Could you check a few things on this model? Use its own coordinates, in mm. A direction names the side the tool comes from. Round coordinates to 2 decimals unless told otherwise and drop trailing zeros. Write each loop counter-clockwise with the first axis right and the second up, starting at its lowest first coordinate (ties: lowest second). Pieces come first, ordered by that corner, then holes. Notation, with made-up numbers: (-40, 47.5) -> (-9, 47.5) arc R21 cw to (-9, 81.5) -> close; hole circle Ø1 at (84, 74.25). An arc over 180 degrees is marked (long way). Answer in a Markdown table with one row per item.
from build123d import *

# Parameters (mm, degrees)
BOSS_EXTRUDE1_DEPTH = 42


with BuildPart() as part:
    # Sketch3 → Boss-Extrude1 (new body)
    with BuildSketch(Plane(origin=(0, 0, 0), x_dir=(0, 0, -1), z_dir=(1, 0, 0))):
        with BuildLine():
            Line((-5.515685425, 6.807463915), (-2.601114729, 3.892893219))
            ThreePointArc((-2.601114729, 3.892893219), (-2.27669138, 3.676120467), (-1.894007948, 3.6))
            Line((-1.894007948, 3.6), (0, 3.6))
            Line((0, 3.6), (0, 2.15))
            ThreePointArc((0, 2.15), (-1.52027958, 1.52027958), (-2.15, 0))
            Line((-2.15, 0), (-3.6, 0))
            Line((-3.6, 0), (-3.6, 1.894007948))
            ThreePointArc((-3.6, 1.894007948), (-3.676120467, 2.27669138), (-3.892893219, 2.601114729))
            Line((-3.892893219, 2.601114729), (-6.807463915, 5.515685425))
            ThreePointArc((-6.807463915, 5.515685425), (-7.679296086, 5.689103626), (-8.17314934, 4.95))
            Line((-8.17314934, 4.95), (-8.17314934, 2.7))
            ThreePointArc((-8.17314934, 2.7), (-8.231727984, 2.558578644), (-8.37314934, 2.5))
            Line((-8.37314934, 2.5), (-9.4, 2.5))
            ThreePointArc((-9.4, 2.5), (-9.824264069, 2.675735931), (-10, 3.1))
            Line((-10, 3.1), (-10, 8.5))
            ThreePointArc((-10, 8.5), (-9.560660172, 9.560660172), (-8.5, 10))
            Line((-8.5, 10), (-3.1, 10))
            ThreePointArc((-3.1, 10), (-2.675735931, 9.824264069), (-2.5, 9.4))
            Line((-2.5, 9.4), (-2.5, 8.37314934))
            ThreePointArc((-2.5, 8.37314934), (-2.558578644, 8.231727984), (-2.7, 8.17314934))
            Line((-2.7, 8.17314934), (-4.95, 8.17314934))
            ThreePointArc((-4.95, 8.17314934), (-5.689103626, 7.679296086), (-5.515685425, 6.807463915))
        make_face()
    extrude(amount=-BOSS_EXTRUDE1_DEPTH)

    # Mirror1: part across plane


with BuildPart() as part_1:
    add(part.part)
    add(part.part.mirror(Plane.ZX))

    # Mirror2: part across plane


with BuildPart() as part_2:
    add(part_1.part)
    add(part_1.part.mirror(Plane.XY))


solid = part_2.part
1) For pin 1 (12 mm diameter, centred on y = 6.5, z = 4, fed in from -X); pin 2 (1 mm diameter, centred on y = 5.5, z = 2.5, fed in from -X); pin 3 (4 mm diameter, centred on x = -29, z = 0, fed in from -Y); pin 4 (1.9 mm diameter, centred on x = -26, z = 1, fed in from +Y), each with a flat end and sliding along its axis, tell me the tip position at first contact or that it passes through.
Findings:
| item | result |
|---|---|
| pin 1 | stops at x = -42 |
| pin 2 | passes through |
| pin 3 | stops at y = -3.61 |
| pin 4 | stops at y = 3.6 |
2) Imagine slicing it at C-C, the plane y = -4.5. Please give me the cut outline in (x, z), plus the area to 3 significant figures.
Findings:
| item | result |
|---|---|
| outline | (-42, -10) -> (0, -10) -> (0, -8.17) -> (-42, -8.17) -> close; (-42, -5.79) -> (0, -5.79) -> (0, -3.21) -> (-42, -3.21) -> close; (-42, 3.21) -> (0, 3.21) -> (0, 5.79) -> (-42, 5.79) -> close; (-42, 8.17) -> (0, 8.17) -> (0, 10) -> (-42, 10) -> close |
| area | 370 mm^2 |
3) Imagine slicing it at A-A, the plane y = 1.25. Please give me the cut outline in (x, z), plus the area to 3 significant figures.
Findings:
| item | result |
|---|---|
| outline | (-42, -3.6) -> (0, -3.6) -> (0, -1.75) -> (-42, -1.75) -> close; (-42, 1.75) -> (0, 1.75) -> (0, 3.6) -> (-42, 3.6) -> close |
| area | 155 mm^2 |
4) Thinking about a two-plate mould opening in Y: for faces 1 (the face through (-21, 6, -10)), 2 (the face through (-21, -10, 6)), 3 (the face through (-20.71, 4.04, 5.33)), which applies, +Y half, -Y half, draft (parallel to the pull), parting line (faces both ways), or undercut?
Findings:
| item | result |
|---|---|
| face 1 | draft |
| face 2 | -Y half |
| face 3 | undercut |
5) Imagine slicing it at B-B, the plane z = -7.75. Please give me the cut outline in (x, y).
Findings:
| item | result |
|---|---|
| outline | (-42, -10) -> (0, -10) -> (0, -5.66) -> (-42, -5.66) -> close; (-42, 5.66) -> (0, 5.66) -> (0, 10) -> (-42, 10) -> close |
6) Please list where these lines run through material, in increasing order: line 1 (Z direction, x = -11.5, y = -8.5); line 2 (Y direction, x = -30, z = -5.5); line 3 (Y direction, x = -22, z = -3.25).
Findings:
| item | result |
|---|---|
| line 1 | z = -10 to -2.5, 2.5 to 10 |
| line 2 | y = -10 to -7.95, -6.79 to -4.21, 4.21 to 6.79, 7.95 to 10 |
| line 3 | y = -10 to -8.17, -4.54 to 4.54, 8.17 to 10 |
7) For faces 4 (the face through (-21, -2.5, 9)), 5 (the face through (-20.706, -5.694, 7.667)), 6 (the face through (-20.71, 9.55, -9.57)), which set-ups out of +Z, -Z, +X, -X, +Y, -Y let a thin tool reach every point of the face, with its end or its side?
Findings:
| item | result |
|---|---|
| face 4 | +Z, +X, -X |
| face 5 | +X, -X |
| face 6 | -Z, +X, -X, +Y |
